Input: dimensioned drawing with shaded views. Units: mm. Origin: part minimum x, y, z. Round coordinates to 2 decimals unless told otherwise and drop trailing zeros. Order: outer loops, then holes, each group sorted by start corner. A loop starts at its lowest first (then second) coordinate and runs counter-clockwise, first axis right, second up. Notation, with made-up numbers: (65.25, 3) - (71.25, 3) arc R30 ccw to (71.25, 28) - close; hole circle Ø11 at (32, 11). An arc over 180 degrees is marked (long way). Put each result on its own line as item: value. Start each with the question number.
(1) Pull-direction query (Z, two-part tool) for the marked faces 1, 2, 3 and 4; classes: released by +Z, released by -Z, zero draft, split by the parting line, or undercut.
(2) Material intervals for L1, parallel to Y at x = 23, z = 2.5; L2, parallel to Z at x = 10, y = 6; L3, parallel to X at y = 2.5, z = 4.25, sorted ascending. Write a range as [from, to].
(3) Section D-D (x = 20). Output: boundary loops of the cut face in (y, z), and give its area (3 significant figures).
(4) Section A-A (x = 23). Output: boundary loops of the cut face in (y, z).
(5) Section C-C (y = 3). Output: boundary loops of the cut face in (x, z).
(6) Section B-B (z = 2.25). Output: boundary loops of the cut face in (x, y).
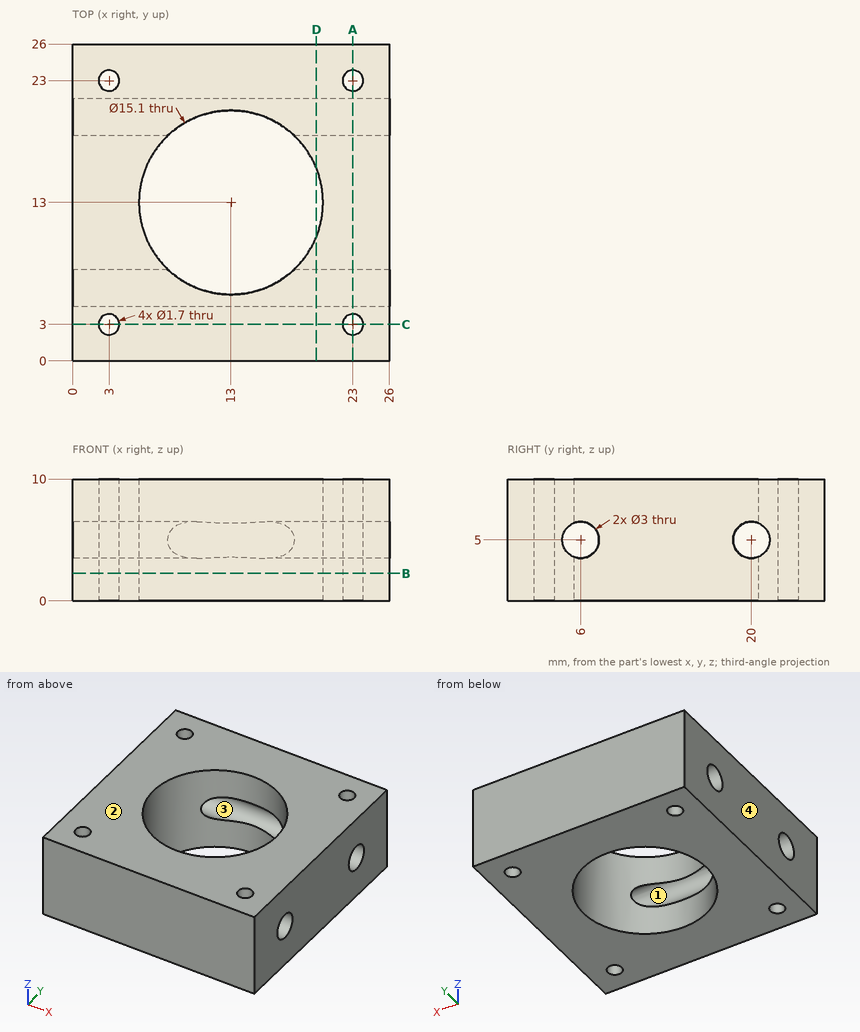
Checks:
1. face 1: undercut
1. face 2: released by +Z
1. face 3: undercut
1. face 4: zero draft
2. L1: y = [0, 2.15], [3.85, 22.15], [23.85, 26]
2. L2: z = [0, 3.5], [6.5, 10]
2. L3: x = [0, 2.31], [3.69, 22.31], [23.69, 26]
3. outline: (0, 0) - (10.17, 0) - (10.17, 10) - (0, 10) - close; (15.83, 0) - (26, 0) - (26, 10) - (15.83, 10) - close; hole circle Ø3 at (6, 5); hole circle Ø3 at (20, 5)
3. area: 189 mm²
4. outline: (0, 0) - (2.15, 0) - (2.15, 10) - (0, 10) - close; (3.85, 0) - (22.15, 0) - (22.15, 10) - (3.85, 10) - close; (23.85, 0) - (26, 0) - (26, 10) - (23.85, 10) - close; hole circle Ø3 at (6, 5); hole circle Ø3 at (20, 5)
5. outline: (0, 0) - (2.15, 0) - (2.15, 10) - (0, 10) - close; (3.85, 0) - (22.15, 0) - (22.15, 10) - (3.85, 10) - close; (23.85, 0) - (26, 0) - (26, 10) - (23.85, 10) - close
6. outline: (0, 0) - (26, 0) - (26, 26) - (0, 26) - close; hole circle Ø1.7 at (3, 3); hole circle Ø1.7 at (3, 23); hole circle Ø15.1 at (13, 13); hole circle Ø1.7 at (23, 3); hole circle Ø1.7 at (23, 23)
